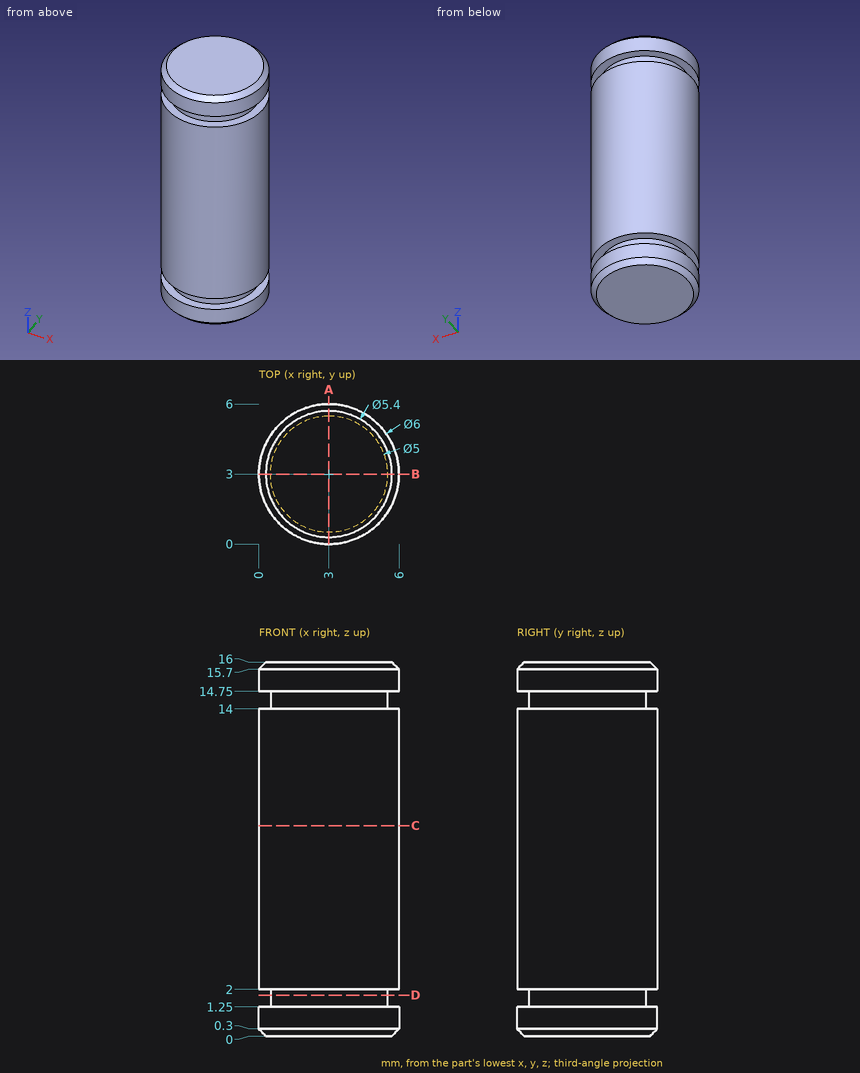
Verification items for this drawing (mm, ordinates from the low corner). Round coordinates to 2 decimals unless told otherwise and drop trailing zeros. Loops run counter-clockwise (first coordinate to the right, second up) from the corner with the lowest first, then second, coordinate; pieces in that order, holes last. Notation, with made-up numbers: (53.25, 72.25) -> (107.25, 72.25) arc R8 ccw to (107.25, 86.25) -> close; hole circle Ø1 at (19.5, -39). An arc over 180 degrees is marked (long way). Write item = value, one per line. Start each with the question number.
1) Gauge pin test, flat end, axial feed: pin 1 Ø3 at (y, z) = (5, 9) entering from +X. Record the tip position at first contact, or that the pin passes through.
2) Thickness scan on probe 1 along Z at (x, y) = (5.65, 3.25); probe 2 along Z at (x, y) = (4.75, 0.65); probe 3 along X at (y, z) = (1.8, 12.75). Record the ranges inside material, lowest first.
3) Sectioned sample at A-A, the plane x = 3. Record the cut outline in (y, z), plus the area to 3 significant figures.
4) Sectioned sample at D-D, the plane z = 1.75. Record the cut outline in (x, y), plus the area to 3 significant figures.
5) Sectioned sample at C-C, the plane z = 9. Record the cut outline in (x, y).
Results are:
q1.pin_1 = 5.96
q2.probe_1 = 0 to 1.25, 2 to 14, 14.75 to 16
q2.probe_2 = 0.23 to 1.25, 2 to 14, 14.75 to 15.77
q2.probe_3 = 0.25 to 5.75
q3.outline = (0, 0.3) -> (0.3, 0) -> (5.7, 0) -> (6, 0.3) -> (6, 1.25) -> (5.5, 1.25) -> (5.5, 2) -> (6, 2) -> (6, 14) -> (5.5, 14) -> (5.5, 14.75) -> (6, 14.75) -> (6, 15.7) -> (5.7, 16) -> (0.3, 16) -> (0, 15.7) -> (0, 14.75) -> (0.5, 14.75) -> (0.5, 14) -> (0, 14) -> (0, 2) -> (0.5, 2) -> (0.5, 1.25) -> (0, 1.25) -> close
q3.area = 94.3 mm^2
q4.outline = circle Ø5 at (3, 3)
q4.area = 19.6 mm^2
q5.outline = circle Ø6 at (3, 3)
